Read the model definition and answer for the solid it produces. Units are mm, in the model's axes. Face numbers are marked on the shaded views. A direction names the side the tool comes from. Coordinates: 2 decimals unless noted, no trailing zeros. Order: outer loops, then holes, each group sorted by start corner. A loop starts at its lowest first (then second) coordinate and runs counter-clockwise, first axis right, second up. Notation, with made-up numbers: (10.25, 76) - (38.25, 76) arc R18 ccw to (38.25, 106) - close; hole circle Ø6 at (-36.75, 17.25). An arc over 180 degrees is marked (long way). Use one line per item in the form item = value.
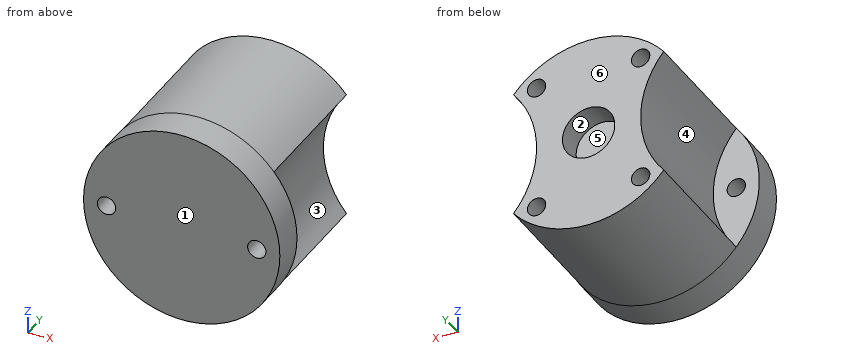
```python
from build123d import *

# Parameters (mm, degrees)
SKETCH073_R     = 15
PAD017_DEPTH    = 5
SKETCH074_R     = 1.4
POCKET046_DEPTH = 5.001
PAD018_DEPTH    = 21.2
SKETCH_R        = 4
POCKET_DEPTH    = 4
SKETCH076_R     = 1.4
POCKET048_DEPTH = 8


with BuildPart() as part:
    # Sketch073 → Pad017 (new body)
    with BuildSketch(Plane.XZ):
        Circle(SKETCH073_R)
    extrude(amount=PAD017_DEPTH)

    # Sketch074 (on Face2 of Pad017) → Pocket046 (cut, through all)
    with BuildSketch(Plane(origin=(0, 0, 0), x_dir=(1, 0, 0), z_dir=(0, 1, 0))):
        with Locations((-11.475, 0)):
            Circle(SKETCH074_R)
        with Locations((11.475, 0)):
            Circle(SKETCH074_R)
    extrude(amount=-POCKET046_DEPTH, mode=Mode.SUBTRACT)

    # Sketch075 (on Face2 of Pocket046) → Pad018 (join)
    with BuildSketch(Plane(origin=(0, 0, 0), x_dir=(1, 0, 0), z_dir=(0, 1, 0))):
        with BuildLine():
            ThreePointArc((11.475, 9.660454), (0, 15), (-11.475, 9.660454))
            ThreePointArc((-11.475, -9.660454), (-7.95, 0), (-11.475, 9.660454))
            ThreePointArc((-11.475, -9.660454), (0, -15), (11.475, -9.660454))
            ThreePointArc((11.475, 9.660454), (7.95, 0), (11.475, -9.660454))
        make_face()
    extrude(amount=PAD018_DEPTH)

    # Sketch (on Face10 of Pad018) → Pocket (cut)
    with BuildSketch(Plane(origin=(0, 21.2, 0), x_dir=(1, 0, 0), z_dir=(0, 1, 0))):
        Circle(SKETCH_R)
    extrude(amount=-POCKET_DEPTH, mode=Mode.SUBTRACT)

    # Sketch076 (on Face10 of Pocket) → Pocket048 (cut)
    with BuildSketch(Plane(origin=(0, 21.2, 0), x_dir=(1, 0, 0), z_dir=(0, 1, 0))):
        with Locations((-7.95, 9.660454)):
            Circle(SKETCH076_R)
        with Locations((7.95, 9.660454)):
            Circle(SKETCH076_R)
        with Locations((-7.95, -9.660454)):
            Circle(SKETCH076_R)
        with Locations((7.95, -9.660454)):
            Circle(SKETCH076_R)
    extrude(amount=-POCKET048_DEPTH, mode=Mode.SUBTRACT)


with BuildPart() as part_1:
    # Body001 placement: moved
    add(part.part.moved(Location((60, -8.4, 60))))


solid = part_1.part
```
(1) Section D-D, the plane x = 70.5 is taken. Write down the section's boundary in (y, z), then the cut area to 3 significant figures.
Answer list:
outline = (-13.4, 49.29) - (12.8, 49.29) - (12.8, 51.63) - (-8.4, 51.63) - (-8.4, 59) - (-13.4, 59) - close; (-13.4, 61) - (-8.4, 61) - (-8.4, 68.37) - (12.8, 68.37) - (12.8, 70.71) - (-13.4, 70.71) - close
area = 197 mm2
(2) Straight lines are drawn through the part: L1, parallel to Z at x = 60, y = 10.5; L2, parallel to X at y = 11.7, z = 60; L3, parallel to Z at x = 67, y = 7.5. For each, find the intervals that lie inside material, in ascending order.
Answer list:
L1 = 45 to 56, 64 to 75
L2 = 52.05 to 56, 64 to 67.95
L3 = 46.73 to 49.31, 51.37 to 68.63, 70.69 to 73.27
(3) Which of the six approach directions +Z, -Z, +X, -X, +Y, -Y give full straight-line access (tool end or side, diameter ignored) to the marked faces 3, 4, 5 and 6?
Answer list:
face_3 = +X, +Y
face_4 = -X, +Y
face_5 = +Y
face_6 = +Z, -Z, +X, -X, +Y
(4) Section B-B, the plane z = 60 is taken. Write down the section's boundary in (x, y) (3 decimals).
Answer list:
outline = (45, -13.4) - (47.125, -13.4) - (47.125, -8.4) - (45, -8.4) - close; (49.925, -13.4) - (70.075, -13.4) - (70.075, -8.4) - (67.95, -8.4) - (67.95, 12.8) - (64, 12.8) - (64, 8.8) - (56, 8.8) - (56, 12.8) - (52.05, 12.8) - (52.05, -8.4) - (49.925, -8.4) - close; (72.875, -13.4) - (75, -13.4) - (75, -8.4) - (72.875, -8.4) - close
(5) Section A-A, the plane y = 7.5 is taken. Write down the section's boundary in (x, z) (3 decimals).
Answer list:
outline = (48.525, 50.34) arc R15 ccw to (71.475, 50.34) arc R15 cw to (71.475, 69.66) arc R15 ccw to (48.525, 69.66) arc R15 cw to start; hole circle Ø2.8 at (52.05, 50.34); hole circle Ø2.8 at (52.05, 69.66); hole circle Ø2.8 at (67.95, 50.34); hole circle Ø2.8 at (67.95, 69.66)
(6) Section C-C, the plane x = 60 is taken. Write down the section's boundary in (y, z).
Answer list:
outline = (-13.4, 45) - (12.8, 45) - (12.8, 56) - (8.8, 56) - (8.8, 64) - (12.8, 64) - (12.8, 75) - (-13.4, 75) - close
(7) The mould has two halves that part along Z. Classify the marked faces 1 and 2: +Z half, -Z half, draft (parallel to the pull), parting line (faces both ways), or undercut.
Answer list:
face_1 = draft
face_2 = undercut
(8) Given pin 1 Ø0.8 at (x, z) = (67.5, 50) entering from +Y; pin 2 Ø1 at (x, z) = (49, 52.5) entering from +Y; pin 3 Ø6 at (y, z) = (2, 55.5) entering from -X; pin 4 Ø12 at (x, y) = (62.5, -3) entering from -Z, each flat-ended and moving along its own axis, determine where each tip first touches the part or whether it passes through.
Answer list:
pin_1 = 4.8
pin_2 = -8.4
pin_3 = 50.04
pin_4 = 45
